Build history of the part. All positions in model axes, mm. Face numbers are marked on the shaded views. A direction names the side the tool comes from. Coordinates: 2 decimals unless noted, no trailing zeros. Loops run counter-clockwise (first coordinate to the right, second up) from the corner with the lowest first, then second, coordinate; pieces in that order, holes last.
Item 1: Cut at D-D (z = 59.5). List the corners of the cut face in (x, y).
Item 2: Cut at C-C (x = 0). List the corners of the cut face in (y, z), and give its area (3 significant figures).
Item 3: Mould opens along Z. For the marked faces 5, 6 and 7 say: released by +Z, released by -Z, zero draft, split by the parting line, or undercut.
Item 4: Cut at B-B (x = 51.5). List the corners of the cut face in (y, z), and give its area (3 significant figures).
Item 5: Flat gauge pins, fed straight in: pin 1 (13.5 mm diameter, centred on y = 24.5, z = 61, fed in from +X); pin 2 (4 mm diameter, centred on x = -95.25, z = 28.575, fed in from +Y); pin 3 (13 mm diameter, centred on y = 13, z = 81, fed in from -X); pin 4 (2 mm diameter, centred on y = 12, z = 45.5, fed in from -X). Where does each tip first touch, or does it go through?
Item 6: Drill centre lines: line 1 along Z through (x, y) = (-95, 31); line 2 along X through (y, z) = (39.5, 3); line 3 along Z through (x, y) = (-28, 7.5). Where is each one in solid material? Low to high.
Item 7: Cut at A-A (x = 95.25). List the corners of the cut face in (y, z), and give its area (3 significant figures).
Item 8: 3-axis set-ups, long thin cutter, end or side, ignore diameter. For the marked faces 1, 2, 3 and 4: which of +Z, -Z, +X, -X, +Y, -Y reach the whole face in a straight line?
from build123d import *

# Parameters (mm, degrees)
BOSS_EXTRUDE1_DEPTH   = 44.45
FILLET1_R             = 6.35
F_8_CLEARANCE_HOLE1_D = 4.4958
FILLET2_R             = 2.54


with BuildPart() as part:
    # Sketch1 → Boss-Extrude1 (new body)
    with BuildSketch(Plane(origin=(0, 0, 0), x_dir=(1, 0, 0), z_dir=(0, 1, 0))):
        Polygon((37.70376, -38.1), (107.95, -38.1), (107.95, 38.1), (-107.95, 38.1), (-107.95, -38.1), (-32.46374, -38.1), (-32.46374, -50.327357955), (25.00376, -50.327357955), (25.00376, -98.262642045), (-32.46374, -98.262642045), (-32.46374, -110.962642045), (37.70376, -110.962642045), align=None)
        Polygon((-76.2, -22.86), (-76.2, 22.86), (-25.4, 7.62), (-25.4, -7.62), align=None, mode=Mode.SUBTRACT)
        Polygon((25.4, -7.62), (25.4, 7.62), (76.2, 22.86), (76.2, -22.86), align=None, mode=Mode.SUBTRACT)
    extrude(amount=BOSS_EXTRUDE1_DEPTH)

    # Fillet1
    fillet1_edges = [part.edges().sort_by_distance(p)[0] for p in [
        (-107.95, 22.225, -38.1),
        (107.95, 22.225, -38.1),
        (107.95, 22.225, 38.1),
        (-107.95, 22.225, 38.1),
        (-76.2, 22.225, -22.86),
        (-76.2, 22.225, 22.86),
        (-25.4, 22.225, 7.62),
        (-25.4, 22.225, -7.62),
        (25.4, 22.225, -7.62),
        (25.4, 22.225, 7.62),
        (76.2, 22.225, 22.86),
        (76.2, 22.225, -22.86),
    ]]
    fillet(fillet1_edges, radius=FILLET1_R)

    # #8 Clearance Hole1 (through all)
    with Locations(Plane(origin=(0, 44.45, 0), x_dir=(1, 0, 0), z_dir=(0, 1, 0))):
        with Locations((95.25, 28.575), (95.25, -28.575), (-95.25, 28.575), (-95.25, -28.575), (0, 0), (-26.11374, -45.4025), (29.76626, -45.4025), (29.76626, -103.1875), (-26.11374, -103.1875)):
            Hole(F_8_CLEARANCE_HOLE1_D / 2)

    # Fillet2
    fillet2_edges = [part.edges().sort_by_distance(p)[0] for p in [
        (37.70376, 22.225, 38.1),
        (37.70376, 22.225, 110.962642045),
        (-32.46374, 22.225, 110.962642045),
        (-32.46374, 22.225, 98.262642045),
        (25.00376, 22.225, 98.262642045),
        (25.00376, 22.225, 50.327357955),
        (-32.46374, 22.225, 50.327357955),
        (-32.46374, 22.225, 38.1),
    ]]
    fillet(fillet2_edges, radius=FILLET2_R)


solid = part.part
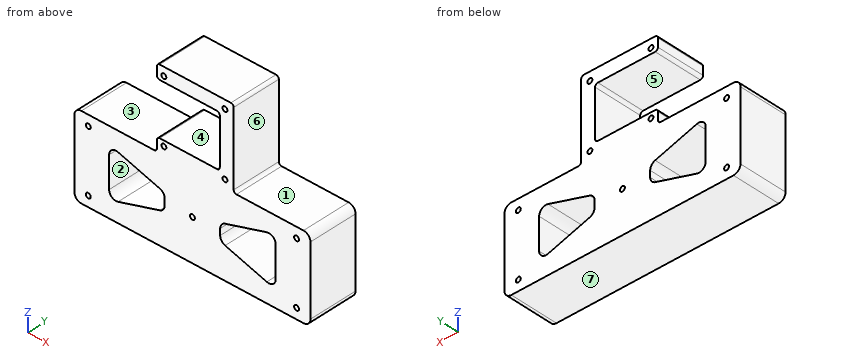
Filled sheet:
1. outline: (25, 0) - (37.7, 0) - (37.7, 44.45) - (25, 44.45) - close
2. outline: (0, -38.1) - (44.45, -38.1) - (44.45, -2.25) - (0, -2.25) - close; (0, 2.25) - (44.45, 2.25) - (44.45, 50.33) - (0, 50.33) - close; (0, 98.26) - (44.45, 98.26) - (44.45, 110.96) - (0, 110.96) - close
2. area: 4,300 mm2
3. face 5: undercut
3. face 6: zero draft
3. face 7: released by -Z
4. outline: (0, -38.1) - (44.45, -38.1) - (44.45, -15.45) - (0, -15.45) - close; (0, 15.45) - (44.45, 15.45) - (44.45, 38.1) - (0, 38.1) - close
4. area: 2,010 mm2
5. pin 1: stops at x = 37.7
5. pin 2: passes through
5. pin 3: stops at x = 25
5. pin 4: stops at x = -32.46
6. line 1: z = -38.1 to -30.81, -26.34 to 26.34, 30.81 to 38.1
6. line 2: x = -107.95 to -76.2, -25.4 to 25.4, 76.2 to 107.95
6. line 3: z = -38.1 to -8.02, 8.02 to 44.18, 46.63 to 50.33, 98.26 to 101.96, 104.41 to 110.96
7. outline: (0, -38.1) - (44.45, -38.1) - (44.45, -30.82) - (0, -30.82) - close; (0, -26.33) - (44.45, -26.33) - (44.45, 26.33) - (0, 26.33) - close; (0, 30.82) - (44.45, 30.82) - (44.45, 38.1) - (0, 38.1) - close
7. area: 2,990 mm2
8. face 1: +Z, +X, +Y, -Y
8. face 2: +Y, -Y
8. face 3: +Z, -X, +Y, -Y
8. face 4: -X, +Y, -Y
